```python
from build123d import *

# Parameters (mm, degrees)
SKETCH_1_R          = 1.55
SKETCH_1_R_2        = 5
EXTRUDE_1_DEPTH     = 3
FILLET_1_R          = 12
SKETCH_2_W          = 5
SKETCH_2_H          = 8
CUT_EXTRUDE_1_DEPTH = 10


with BuildPart() as part:
    # 草图1 → 凸台-拉伸1 (new body)
    with BuildSketch(Plane.XY):
        Polygon((-29.5, 32), (103.4, 32), (103.4, 7), (103.4, 4.5), (88.9, -10), (86.4, -10), (61.4, -10), (58.9, -10), (50.9, -2), (23, -2), (15, -10), (12.5, -10), (-12.5, -10), (-15, -10), (-29.5, 4.5), (-29.5, 7), align=None)
        with Locations((-7.5, 4)):
            Circle(SKETCH_1_R, mode=Mode.SUBTRACT)
        with Locations((-7.5, -4)):
            Circle(SKETCH_1_R, mode=Mode.SUBTRACT)
        with Locations((7.5, -4)):
            Circle(SKETCH_1_R, mode=Mode.SUBTRACT)
        with Locations((7.5, 4)):
            Circle(SKETCH_1_R, mode=Mode.SUBTRACT)
        with Locations((66.4, 4)):
            Circle(SKETCH_1_R, mode=Mode.SUBTRACT)
        with Locations((66.4, -4)):
            Circle(SKETCH_1_R, mode=Mode.SUBTRACT)
        with Locations((81.4, 4)):
            Circle(SKETCH_1_R, mode=Mode.SUBTRACT)
        with Locations((81.4, -4)):
            Circle(SKETCH_1_R, mode=Mode.SUBTRACT)
        with Locations((-24.5, 27)):
            Circle(SKETCH_1_R, mode=Mode.SUBTRACT)
        with Locations((-24.5, 12)):
            Circle(SKETCH_1_R, mode=Mode.SUBTRACT)
        with Locations((16.95, 19.5)):
            Circle(SKETCH_1_R, mode=Mode.SUBTRACT)
        with Locations((36.95, 27)):
            Circle(SKETCH_1_R, mode=Mode.SUBTRACT)
        with Locations((36.95, 12)):
            Circle(SKETCH_1_R, mode=Mode.SUBTRACT)
        with Locations((56.95, 19.5)):
            Circle(SKETCH_1_R, mode=Mode.SUBTRACT)
        with Locations((96.95, 27)):
            Circle(SKETCH_1_R, mode=Mode.SUBTRACT)
        with Locations((96.95, 12)):
            Circle(SKETCH_1_R, mode=Mode.SUBTRACT)
        with Locations((-23.05, 19.5)):
            Circle(SKETCH_1_R, mode=Mode.SUBTRACT)
        with Locations((36.95, 2)):
            Circle(SKETCH_1_R, mode=Mode.SUBTRACT)
        with Locations((73.9, 13.5)):
            Circle(SKETCH_1_R, mode=Mode.SUBTRACT)
        with Locations((70.4, 21.5)):
            Circle(SKETCH_1_R, mode=Mode.SUBTRACT)
        with Locations(Location((77.4, 21.5, 0), (0, 0, 180))):
            Circle(SKETCH_1_R, mode=Mode.SUBTRACT)
        with Locations((0, 13.5)):
            Circle(SKETCH_1_R, mode=Mode.SUBTRACT)
        with Locations((-3.5, 21.5)):
            Circle(SKETCH_1_R, mode=Mode.SUBTRACT)
        with Locations((3.5, 21.5)):
            Circle(SKETCH_1_R, mode=Mode.SUBTRACT)
        with Locations((-20, -0.5)):
            Circle(SKETCH_1_R, mode=Mode.SUBTRACT)
        with Locations(Location((93.9, -0.5, 0), (0, 0, 180))):
            Circle(SKETCH_1_R, mode=Mode.SUBTRACT)
        with Locations(Location((20, -0.5, 0), (0, 0, 180))):
            Circle(SKETCH_1_R, mode=Mode.SUBTRACT)
        with Locations((53.9, -0.5)):
            Circle(SKETCH_1_R, mode=Mode.SUBTRACT)
        Circle(SKETCH_1_R, mode=Mode.SUBTRACT)
        with Locations((73.9, 0)):
            Circle(SKETCH_1_R, mode=Mode.SUBTRACT)
        with Locations((-10, 12.5)):
            Circle(SKETCH_1_R_2, mode=Mode.SUBTRACT)
        with Locations(Location((83.9, 12.5, 0), (0, 0, 180))):
            Circle(SKETCH_1_R_2, mode=Mode.SUBTRACT)
        with Locations(Location((10, 12.5, 0), (0, 0, 180))):
            Circle(SKETCH_1_R_2, mode=Mode.SUBTRACT)
        with Locations((63.9, 12.5)):
            Circle(SKETCH_1_R_2, mode=Mode.SUBTRACT)
        with BuildLine():
            Line((-15.05, 29), (0.95, 29))
            ThreePointArc((0.95, 29), (2.95, 27), (0.95, 25))
            Line((0.95, 25), (-15.05, 25))
            ThreePointArc((-15.05, 25), (-17.05, 27), (-15.05, 29))
        make_face(mode=Mode.SUBTRACT)
        with BuildLine():
            Line((12.95, 29), (28.95, 29))
            ThreePointArc((28.95, 29), (30.95, 27), (28.95, 25))
            Line((28.95, 25), (12.95, 25))
            ThreePointArc((12.95, 25), (10.95, 27), (12.95, 29))
        make_face(mode=Mode.SUBTRACT)
        with BuildLine():
            Line((44.95, 29), (60.95, 29))
            ThreePointArc((60.95, 29), (62.95, 27), (60.95, 25))
            Line((60.95, 25), (44.95, 25))
            ThreePointArc((44.95, 25), (42.95, 27), (44.95, 29))
        make_face(mode=Mode.SUBTRACT)
        with BuildLine():
            Line((72.95, 29), (88.95, 29))
            ThreePointArc((88.95, 29), (90.95, 27), (88.95, 25))
            Line((88.95, 25), (72.95, 25))
            ThreePointArc((72.95, 25), (70.95, 27), (72.95, 29))
        make_face(mode=Mode.SUBTRACT)
        with BuildLine():
            Line((23.5, 12.5), (23.5, 5))
            ThreePointArc((23.5, 5), (21, 2.5), (18.5, 5))
            Line((18.5, 5), (18.5, 12.5))
            ThreePointArc((18.5, 12.5), (21, 15), (23.5, 12.5))
        make_face(mode=Mode.SUBTRACT)
        with BuildLine():
            Line((32.45, 12.5), (32.45, 5))
            ThreePointArc((32.45, 5), (29.95, 2.5), (27.45, 5))
            Line((27.45, 5), (27.45, 12.5))
            ThreePointArc((27.45, 12.5), (29.95, 15), (32.45, 12.5))
        make_face(mode=Mode.SUBTRACT)
        with BuildLine():
            Line((50.4, 12.5), (50.4, 5))
            ThreePointArc((50.4, 5), (52.9, 2.5), (55.4, 5))
            Line((55.4, 5), (55.4, 12.5))
            ThreePointArc((55.4, 12.5), (52.9, 15), (50.4, 12.5))
        make_face(mode=Mode.SUBTRACT)
        with BuildLine():
            Line((41.45, 12.5), (41.45, 5))
            ThreePointArc((41.45, 5), (43.95, 2.5), (46.45, 5))
            Line((46.45, 5), (46.45, 12.5))
            ThreePointArc((46.45, 12.5), (43.95, 15), (41.45, 12.5))
        make_face(mode=Mode.SUBTRACT)
    extrude(amount=EXTRUDE_1_DEPTH)

    # 圆角1
    fillet_1_edges = [part.edges().sort_by_distance(p)[0] for p in [
        (50.9, -2, 1.5),
        (23, -2, 1.5),
    ]]
    fillet(fillet_1_edges, radius=FILLET_1_R)

    # 草图2 → 切除-拉伸1 (cut)
    with BuildSketch(Plane.XY.offset(3)):
        with Locations((-10, -12)):
            Rectangle(SKETCH_2_W, SKETCH_2_H)
        with Locations((10, -12)):
            Rectangle(SKETCH_2_W, SKETCH_2_H)
        with Locations((83.9, -12)):
            Rectangle(SKETCH_2_W, SKETCH_2_H)
        with Locations((63.9, -12)):
            Rectangle(SKETCH_2_W, SKETCH_2_H)
    extrude(amount=-CUT_EXTRUDE_1_DEPTH, mode=Mode.SUBTRACT)


solid = part.part
```
CAD build for the part. Positions are in the model's coordinates, mm. A direction names the side the tool comes from. Round coordinates to 2 decimals unless told otherwise and drop trailing zeros. Loops run counter-clockwise (first coordinate to the right, second up) from the corner with the lowest first, then second, coordinate; pieces in that order, holes last. Notation, with made-up numbers: M 49,51.25 L 70,51.25 A15 cw 70,75.25 Z; hole C 63,86 d3. An arc over 180 degrees is marked long. Return JSON: item names as keys, results as strings. Group by question number.
(1) Saw through at C-C, the plane x = 96.95. List the corners of the cut face in (y, z).
(2) Tool access for faces 4 (the flat face through (64, -8, 2)), 5 (the cylindrical face through (52.8, 2.5, 1.5)), 6 (the flat face through (38, 16, 0)): list every direction of +Z, -Z, +X, -X, +Y, -Y with a clear straight run to the whole face (end or side of a thin tool).
(3) Saw through at A-A, the plane y = 27. Give the number of separate pieces and of enclosed holes in the cut face, and give its area (3 significant figures).
(4) Wall check: probe 1 along Y at (x, z) = (36.95, 1.3); probe 2 along Y at (x, z) = (-3.5, 1.7); probe 3 along X at (y, z) = (6, 2.5). Give the ranges that are in metal, low to high. Write a range as [from, to].
(5) Saw through at B-B, the plane x = -20. List the corners of the cut face in (y, z), and give its area (3 significant figures).
(6) Mould opens along Y. For faces 1 (the flat face through (81, 29, 1)), 2 (the flat face through (38, 16, 3)), 3 (the flat face through (14, -10, 1)) say: +Y half, -Y half, draft (parallel to the pull), parting line (faces both ways), or undercut.
Answer list:
{
 "1": {"outline": "M -1.95,0 L 10.45,0 L 10.45,3 L -1.95,3 Z; M 13.55,0 L 25.45,0 L 25.45,3 L 13.55,3 Z; M 28.55,0 L 32,0 L 32,3 L 28.55,3 Z"},
 "2": {"face 4": "+Z, -Z, -Y", "face 5": "+Z, -Z", "face 6": "-Z, +X, -X, +Y, -Y"},
 "3": {"separate pieces": "8", "enclosed holes": "0", "area": "131 mm2"},
 "4": {"probe 1": "[-2, 0.45], [3.55, 10.45], [13.55, 25.45], [28.55, 32]", "probe 2": "[-10, 19.95], [23.05, 25], [29, 32]", "probe 3": "[-29.5, 18.5], [23.5, 27.45], [32.45, 41.45], [46.45, 50.4], [55.4, 103.4]"},
 "5": {"outline": "M -5,0 L -2.05,0 L -2.05,3 L -5,3 Z; M 1.05,0 L 32,0 L 32,3 L 1.05,3 Z", "area": "102 mm2"},
 "6": {"face 1": "undercut", "face 2": "draft", "face 3": "-Y half"}
}
